Model file for the job. Use its own axes, mm. Face numbers are marked on the shaded views. Coordinates: 2 decimals unless noted, no trailing zeros. Write each loop counter-clockwise with the first axis right and the second up, starting at its lowest first coordinate (ties: lowest second). Pieces come first, ordered by that corner, then holes. Notation, with made-up numbers: (68, 69.25) -> (76, 69.25) arc R8 ccw to (76, 82.25) -> close; hole circle Ø9 at (-5.75, 41). An arc over 180 degrees is marked (long way). Answer as a JSON object with one key per item and string values. Group by question number.
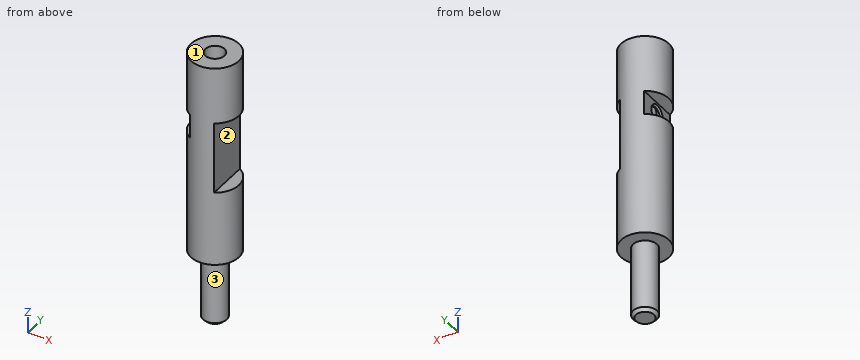
from build123d import *

# Parameters (mm, degrees)
SKETCH1_R                       = 2
BOSS_EXTRUDE1_DEPTH             = 12
CHAMFER1_SIZE                   = 0.5
SKETCH2_R                       = 4
BOSS_EXTRUDE2_DEPTH             = 34
SKETCH3_R                       = 1.6
CUT_EXTRUDE1_DEPTH              = 14
CUT_EXTRUDE2_DEPTH              = 47.346520905
CUT_EXTRUDE2_DEPTH_BACK         = 47.346520905
SKETCH4_W                       = 2
SKETCH4_H                       = 12
M3X0_5_TAPPED_HOLE1_D           = 2.5
M3X0_5_TAPPED_HOLE1_DEPTH       = 13.248924226
M3X0_5_TAPPED_HOLE1_CSINK_D     = 3.05
M3X0_5_TAPPED_HOLE1_CSINK_ANGLE = 90
M3X0_5_TAPPED_HOLE1_TIP         = 0.751075774
CUT_EXTRUDE3_DEPTH              = 47.346520905
CUT_EXTRUDE3_DEPTH_BACK         = 47.346520905
SKETCH7_W                       = 2
SKETCH7_H                       = 4
M3X0_5_TAPPED_HOLE3_D           = 2.5
M3X0_5_TAPPED_HOLE3_DEPTH       = 1.248924226
M3X0_5_TAPPED_HOLE3_CSINK_D     = 3.05
M3X0_5_TAPPED_HOLE3_CSINK_ANGLE = 90
M3X0_5_TAPPED_HOLE3_TIP         = 0.751075774


with BuildPart() as part:
    # Sketch1 → Boss-Extrude1 (new body)
    with BuildSketch(Plane.XY):
        Circle(SKETCH1_R)
    extrude(amount=BOSS_EXTRUDE1_DEPTH)

    # Chamfer1
    chamfer1_edges = [part.edges().sort_by_distance(p)[0] for p in [
        (-2, 0, 0),
    ]]
    chamfer(chamfer1_edges, length=CHAMFER1_SIZE)

    # Sketch2 → Boss-Extrude2 (add)
    with BuildSketch(Plane.XY.offset(12)):
        Circle(SKETCH2_R)
    extrude(amount=BOSS_EXTRUDE2_DEPTH)

    # Sketch3 → Cut-Extrude1 (cut)
    with BuildSketch(Plane.XY.offset(46)):
        Circle(SKETCH3_R)
    extrude(amount=-CUT_EXTRUDE1_DEPTH, mode=Mode.SUBTRACT)

    # Sketch4 → Cut-Extrude2 (cut, two sides: drawn at the far end of the back side and taken through both)
    with BuildSketch(Plane(origin=(0, 0, 0), x_dir=(1, 0, 0), z_dir=(0, 1, 0)).offset(-CUT_EXTRUDE2_DEPTH_BACK)):
        with Locations((3, -30.5)):
            Rectangle(SKETCH4_W, SKETCH4_H)
    extrude(amount=CUT_EXTRUDE2_DEPTH + CUT_EXTRUDE2_DEPTH_BACK, mode=Mode.SUBTRACT)

    # M3x0.5 Tapped Hole1
    with Locations(Plane.XY.offset(46)):
        with Locations((0, 0)):
            CounterSinkHole(M3X0_5_TAPPED_HOLE1_D / 2, M3X0_5_TAPPED_HOLE1_CSINK_D / 2, depth=M3X0_5_TAPPED_HOLE1_DEPTH, counter_sink_angle=M3X0_5_TAPPED_HOLE1_CSINK_ANGLE)
            with Locations((0, 0, -(M3X0_5_TAPPED_HOLE1_DEPTH + M3X0_5_TAPPED_HOLE1_TIP / 2))):  # 118° drill point
                Cone(0, M3X0_5_TAPPED_HOLE1_D / 2, M3X0_5_TAPPED_HOLE1_TIP, mode=Mode.SUBTRACT)

    # Sketch7 → Cut-Extrude3 (cut, two sides: drawn at the far end of the back side and taken through both)
    with BuildSketch(Plane(origin=(0, 0, 0), x_dir=(1, 0, 0), z_dir=(0, 1, 0)).offset(-CUT_EXTRUDE3_DEPTH_BACK)):
        with Locations((-3, -34.5)):
            Rectangle(SKETCH7_W, SKETCH7_H)
    extrude(amount=CUT_EXTRUDE3_DEPTH + CUT_EXTRUDE3_DEPTH_BACK, mode=Mode.SUBTRACT)

    # M3x0.5 Tapped Hole3
    with Locations(Plane(origin=(-2, -0.015660655, 34.578358954), x_dir=(0, 0, -1), z_dir=(-1, 0, 0))):
        with Locations((0, 0)):
            CounterSinkHole(M3X0_5_TAPPED_HOLE3_D / 2, M3X0_5_TAPPED_HOLE3_CSINK_D / 2, depth=M3X0_5_TAPPED_HOLE3_DEPTH, counter_sink_angle=M3X0_5_TAPPED_HOLE3_CSINK_ANGLE)
            with Locations((0, 0, -(M3X0_5_TAPPED_HOLE3_DEPTH + M3X0_5_TAPPED_HOLE3_TIP / 2))):  # 118° drill point
                Cone(0, M3X0_5_TAPPED_HOLE3_D / 2, M3X0_5_TAPPED_HOLE3_TIP, mode=Mode.SUBTRACT)


solid = part.part
(1) Cut at C-C on z = 38. List the corners of the cut face in (x, y), plus the area to 3 significant figures.
(2) Pin check, flat tips, straight feed: pin 1 (1 mm diameter, centred on x = -2.5, y = -0.5, fed in from -Z); pin 2 (4 mm diameter, centred on x = 1, z = 9, fed in from -Y); pin 3 (4 mm diameter, centred on x = -2.5, z = 28, fed in from +Y). Stop position of each tip, or through.
(3) Wall check: probe 1 along Y at (x, z) = (0, 41); probe 2 along Z at (x, y) = (3, -1.75); probe 3 along Z at (x, y) = (1.75, 1.75). Give the ranges that are in metal, low to high.
(4) Pull direction Z, two halves, no side cores. Call the marked faces 1, 2 and 3: released by +Z, released by -Z, zero draft, split by the parting line, or undercut.
(5) Cut at D-D on z = 6. List the corners of the cut face in (x, y).
(6) Cut at A-A on x = 0. List the corners of the cut face in (y, z), plus the area to 3 significant figures.
(7) Cut at B-B on y = -2.5. List the corners of the cut face in (x, z).
Results found:
{
 "1": {"outline": "circle Ø8 at (0, 0); hole circle Ø3.2 at (0, 0)", "area": "42.2 mm²"},
 "2": {"pin 1": "stops at z = 12", "pin 2": "stops at y = -2", "pin 3": "stops at y = 3.97"},
 "3": {"probe 1": "y = -4 to -1.6, 1.6 to 4", "probe 2": "z = 12 to 24.5, 36.5 to 46", "probe 3": "z = 12 to 46"},
 "4": {"face 1": "released by +Z", "face 2": "undercut", "face 3": "zero draft"},
 "5": {"outline": "circle Ø4 at (0, 0)"},
 "6": {"outline": "(-4, 12) -> (-2, 12) -> (-2, 0.5) -> (-1.5, 0) -> (1.5, 0) -> (2, 0.5) -> (2, 12) -> (4, 12) -> (4, 46) -> (1.6, 46) -> (1.6, 32) -> (-1.6, 32) -> (-1.6, 46) -> (-4, 46) -> close", "area": "275 mm²"},
 "7": {"outline": "(-3.12, 12) -> (3.12, 12) -> (3.12, 24.5) -> (2, 24.5) -> (2, 36.5) -> (3.12, 36.5) -> (3.12, 46) -> (-3.12, 46) -> (-3.12, 36.5) -> (-2, 36.5) -> (-2, 32.5) -> (-3.12, 32.5) -> close"}
}
